from build123d import *

# Parameters (mm, degrees)
F0_R     = 1.5
F0_R_2   = 1.25
F1_DEPTH = 1.5
F2_DEPTH = 8
F3_R     = 2
F4_R     = 2


with BuildPart() as f1:
    # F0 (on Top) → F1 (new body)
    with BuildSketch(Plane.XY):
        with BuildLine():
            Line((-13.304709, -19), (13.2, -19))
            Line((13.2, -19), (13.2, -15.25))
            ThreePointArc((13.2, -15.25), (13.800431, -13.800431), (15.25, -13.2))
            Line((15.25, -13.2), (19, -13.2))
            Line((19, -13.2), (19, 13.654472))
            Line((19, 13.654472), (15.25, 13.654472))
            ThreePointArc((15.25, 13.654472), (13.800431, 14.254903), (13.2, 15.704472))
            Line((13.2, 15.704472), (13.2, 19))
            Line((13.2, 19), (-13.2, 19))
            Line((-13.2, 19), (-13.2, 15.25))
            ThreePointArc((-13.2, 15.25), (-13.800431, 13.800431), (-15.25, 13.2))
            Line((-15.25, 13.2), (-19, 13.2))
            Line((-19, 13.2), (-19, -13.2))
            Line((-19, -13.2), (-15.25, -13.2))
            ThreePointArc((-15.25, -13.2), (-13.780186, -13.820963), (-13.200811, -15.307662))
            Line((-13.200811, -15.307662), (-13.304709, -19))
        make_face()
        with BuildLine():
            Line((-16.5, -19), (-13.304709, -19))
            Line((-13.304709, -19), (-13.200811, -15.307662))
            ThreePointArc((-13.200811, -15.307662), (-13.780186, -13.820963), (-15.25, -13.2))
            Line((-15.25, -13.2), (-19, -13.2))
            Line((-19, -13.2), (-19, -16.5))
            ThreePointArc((-19, -16.5), (-18.267767, -18.267767), (-16.5, -19))
        make_face()
        with Locations((-15.25, -15.25)):
            Circle(F0_R, mode=Mode.SUBTRACT)
        with BuildLine():
            Line((13.2, -19), (16, -19))
            ThreePointArc((16, -19), (18.12132, -18.12132), (19, -16))
            Line((19, -16), (19, -13.2))
            Line((19, -13.2), (15.25, -13.2))
            ThreePointArc((15.25, -13.2), (13.800431, -13.800431), (13.2, -15.25))
            Line((13.2, -15.25), (13.2, -19))
        make_face()
        with Locations((15.25, -15.25)):
            Circle(F0_R_2, mode=Mode.SUBTRACT)
        with BuildLine():
            Line((15.25, 13.654472), (19, 13.654472))
            Line((19, 13.654472), (19, 16))
            ThreePointArc((19, 16), (18.12132, 18.12132), (16, 19))
            Line((16, 19), (13.2, 19))
            Line((13.2, 19), (13.2, 15.704472))
            ThreePointArc((13.2, 15.704472), (13.800431, 14.254903), (15.25, 13.654472))
        make_face()
        with Locations((15.25, 15.704472)):
            Circle(F0_R_2, mode=Mode.SUBTRACT)
        with BuildLine():
            Line((-19, 16), (-19, 13.2))
            Line((-19, 13.2), (-15.25, 13.2))
            ThreePointArc((-15.25, 13.2), (-13.800431, 13.800431), (-13.2, 15.25))
            Line((-13.2, 15.25), (-13.2, 19))
            Line((-13.2, 19), (-16, 19))
            ThreePointArc((-16, 19), (-18.12132, 18.12132), (-19, 16))
        make_face()
        with Locations((-15.25, 15.25)):
            Circle(F0_R_2, mode=Mode.SUBTRACT)
    extrude(amount=F1_DEPTH)

    # F0 (on Top) → F2 (join)
    with BuildSketch(Plane.XY):
        with BuildLine():
            Line((-16.5, -19), (-13.304709, -19))
            Line((-13.304709, -19), (-13.200811, -15.307662))
            ThreePointArc((-13.200811, -15.307662), (-13.780186, -13.820963), (-15.25, -13.2))
            Line((-15.25, -13.2), (-19, -13.2))
            Line((-19, -13.2), (-19, -16.5))
            ThreePointArc((-19, -16.5), (-18.267767, -18.267767), (-16.5, -19))
        make_face()
        with Locations((-15.25, -15.25)):
            Circle(F0_R, mode=Mode.SUBTRACT)
        with BuildLine():
            Line((13.2, -19), (16, -19))
            ThreePointArc((16, -19), (18.12132, -18.12132), (19, -16))
            Line((19, -16), (19, -13.2))
            Line((19, -13.2), (15.25, -13.2))
            ThreePointArc((15.25, -13.2), (13.800431, -13.800431), (13.2, -15.25))
            Line((13.2, -15.25), (13.2, -19))
        make_face()
        with Locations((15.25, -15.25)):
            Circle(F0_R_2, mode=Mode.SUBTRACT)
        with BuildLine():
            Line((15.25, 13.654472), (19, 13.654472))
            Line((19, 13.654472), (19, 16))
            ThreePointArc((19, 16), (18.12132, 18.12132), (16, 19))
            Line((16, 19), (13.2, 19))
            Line((13.2, 19), (13.2, 15.704472))
            ThreePointArc((13.2, 15.704472), (13.800431, 14.254903), (15.25, 13.654472))
        make_face()
        with Locations((15.25, 15.704472)):
            Circle(F0_R_2, mode=Mode.SUBTRACT)
        with BuildLine():
            Line((-19, 16), (-19, 13.2))
            Line((-19, 13.2), (-15.25, 13.2))
            ThreePointArc((-15.25, 13.2), (-13.800431, 13.800431), (-13.2, 15.25))
            Line((-13.2, 15.25), (-13.2, 19))
            Line((-13.2, 19), (-16, 19))
            ThreePointArc((-16, 19), (-18.12132, 18.12132), (-19, 16))
        make_face()
        with Locations((-15.25, 15.25)):
            Circle(F0_R_2, mode=Mode.SUBTRACT)
    extrude(amount=F2_DEPTH)

    # F3
    f3_edges = [f1.edges().sort_by_distance(p)[0] for p in [
        (-19, 13.2, 4.75),
    ]]
    fillet(f3_edges, radius=F3_R)

    # F4
    f4_edges = [f1.edges().sort_by_distance(p)[0] for p in [
        (-13.2, 19, 4.75),
        (13.2, 19, 4.75),
        (19, 13.654472, 4.75),
        (19, -13.2, 4.75),
        (13.2, -19, 4.75),
        (-13.304709, -19, 4.75),
        (-19, -13.2, 4.75),
    ]]
    fillet(f4_edges, radius=F4_R)


solid = f1.part
Source: CAD feature listing. Evaluate the final solid. Frame: model axes, mm. A direction names the side the tool comes from. Give positions to 0.01 mm unless a question says otherwise; leave off trailing zeros. Order: outer loops, then holes, each group sorted by start corner. A loop starts at its lowest first (then second) coordinate and runs counter-clockwise, first axis right, second up. Notation, with made-up numbers: (60, -38.5) -> (91, -38.5) arc R25 ccw to (91, -4.5) -> close; hole circle Ø5 at (20, 81.5). An arc over 180 degrees is marked (long way). Write item = value, one per line.
Item 1: Section query A-A (z = 4.25). State how many separate pieces and enclosed holes the cut face has, then the cut area to 3 significant figures.
Check result:
separate_pieces = 4
enclosed_holes = 4
area = 92.4 mm²
Item 2: Ray query, probe 1 along Y at (x, z) = (-15.25, 5.5); probe 2 along Y at (x, z) = (15.25, 3); probe 3 along X at (y, z) = (16, 7.25). Return the intervals inside material, ascending.
Check result:
probe_1 = -19 to -16.75, -13.75 to -13.2, 13.2 to 14, 16.5 to 19
probe_2 = -19 to -16.5, -14 to -13.2, 13.65 to 14.45, 16.95 to 19
probe_3 = -19 to -16.25, -14.25 to -13.2, 13.2 to 14.04, 16.46 to 19
Item 3: Set-up query: faces 1 (the face through (13.2, -16, 5)), 2 (the face through (16, 13.654, 5)), 3 (the face through (0, 0, 1.5)). Return all of +Z, -Z, +X, -X, +Y, -Y with unobstructed straight access to the full face (end or side cutting, diameter ignored); none if empty.
Check result:
face_1 = +Z, +Y, -Y
face_2 = +Z, +X
face_3 = +Z
Item 4: Contact query for flat-ended pins moving along their axis: pin 1 (12 mm diameter, centred on x = -10.5, y = -2.5, fed in from +Z); pin 2 (3 mm diameter, centred on x = 10.5, y = 0, fed in from -Z); pin 3 (3 mm diameter, centred on y = 13.5, z = 4.5, fed in from -X); pin 4 (0.5 mm diameter, centred on x = 16.5, z = 5.5, fed in from +Y). Output: stop coordinate, or through.
Check result:
pin_1 = 1.5
pin_2 = 0
pin_3 = -18.99
pin_4 = 18.99
Item 5: Section query B-B (y = -1.5). Output: boundary loops of the cut face in (x, z).
Check result:
outline = (-19, 0) -> (19, 0) -> (19, 1.5) -> (-19, 1.5) -> close
Item 6: Mould query, pull axis Y, two halves, no side actions, for faces 4 (the face through (19, -2, 1)), 5 (the face through (13.77, -18.4, 4.8)), 6 (the face through (18.43, -13.8, 4.8)). Classes: +Y half, -Y half, draft (parallel to the pull), parting line (faces both ways), or undercut.
Check result:
face_4 = draft
face_5 = -Y half
face_6 = undercut
